from build123d import *

# Parameters (mm, degrees)
SKETCH1_R           = 0.5
BOSS_EXTRUDE1_DEPTH = 3
BOSS_EXTRUDE2_DEPTH = 3


with BuildPart() as part:
    # Sketch1 → Boss-Extrude1 (new body)
    with BuildSketch(Plane(origin=(0, 0, 0), x_dir=(1, 0, 0), z_dir=(0, 1, 0))):
        with BuildLine():
            Line((50, 20), (-50, 20))
            ThreePointArc((-50, 20), (-70, 0), (-50, -20))
            Line((-50, -20), (50, -20))
            ThreePointArc((50, -20), (70, 0), (50, 20))
        make_face()
        with Locations(Location((-48.85, -16.15, 0), (0, 0, 270))):
            Circle(SKETCH1_R, mode=Mode.SUBTRACT)
        with BuildLine():
            ThreePointArc((-48.85, -12.65), (-48.35, -13.15), (-48.85, -13.65))
            ThreePointArc((-48.85, -13.65), (-49.35, -13.15), (-48.85, -12.65))
        make_face(mode=Mode.SUBTRACT)
        with BuildLine():
            ThreePointArc((-48.85, -9.65), (-48.35, -10.15), (-48.85, -10.65))
            ThreePointArc((-48.85, -10.65), (-49.35, -10.15), (-48.85, -9.65))
        make_face(mode=Mode.SUBTRACT)
        Polygon((-30, -10), (-30, 8.197224362), (-16.352081728, -0.901387819), align=None, mode=Mode.SUBTRACT)
        Polygon((-2.704163457, -10), (-24.591673087, -10), (-13.647918272, -2.704163457), align=None, mode=Mode.SUBTRACT)
        with Locations(Location((48.85, -16.15, 0), (0, 0, 270))):
            Circle(SKETCH1_R, mode=Mode.SUBTRACT)
        with BuildLine():
            ThreePointArc((48.85, -12.65), (49.35, -13.15), (48.85, -13.65))
            ThreePointArc((48.85, -13.65), (48.35, -13.15), (48.85, -12.65))
        make_face(mode=Mode.SUBTRACT)
        with BuildLine():
            ThreePointArc((48.85, -9.65), (49.35, -10.15), (48.85, -10.65))
            ThreePointArc((48.85, -10.65), (48.35, -10.15), (48.85, -9.65))
        make_face(mode=Mode.SUBTRACT)
        Polygon((24.591673087, -10), (2.704163457, -10), (13.647918272, -2.704163457), align=None, mode=Mode.SUBTRACT)
        Polygon((30, 8.197224362), (30, -10), (16.352081728, -0.901387819), align=None, mode=Mode.SUBTRACT)
        with Locations(Location((-65, 0, 0), (0, 0, 270))):
            Circle(SKETCH1_R, mode=Mode.SUBTRACT)
        with Locations(Location((-62, 0, 0), (0, 0, 270))):
            Circle(SKETCH1_R, mode=Mode.SUBTRACT)
        with Locations(Location((-59, 0, 0), (0, 0, 270))):
            Circle(SKETCH1_R, mode=Mode.SUBTRACT)
        with BuildLine():
            ThreePointArc((-44.85, 0), (-46.021572875, -2.828427125), (-48.85, -4))
            ThreePointArc((-48.85, -4), (-52.85, 0), (-48.85, 4))
            ThreePointArc((-48.85, 4), (-46.021572875, 2.828427125), (-44.85, 0))
        make_face(mode=Mode.SUBTRACT)
        with BuildLine():
            ThreePointArc((-38.2, 0), (-38.7, -0.5), (-39.2, 0))
            ThreePointArc((-39.2, 0), (-38.7, 0.5), (-38.2, 0))
        make_face(mode=Mode.SUBTRACT)
        with BuildLine():
            ThreePointArc((-35.2, 0), (-35.7, -0.5), (-36.2, 0))
            ThreePointArc((-36.2, 0), (-35.7, 0.5), (-35.2, 0))
        make_face(mode=Mode.SUBTRACT)
        with Locations(Location((-32.7, 0, 0), (0, 0, 270))):
            Circle(SKETCH1_R, mode=Mode.SUBTRACT)
        with BuildLine():
            ThreePointArc((-48.85, 10.65), (-48.35, 10.15), (-48.85, 9.65))
            ThreePointArc((-48.85, 9.65), (-49.35, 10.15), (-48.85, 10.65))
        make_face(mode=Mode.SUBTRACT)
        with BuildLine():
            ThreePointArc((-48.85, 13.65), (-48.35, 13.15), (-48.85, 12.65))
            ThreePointArc((-48.85, 12.65), (-49.35, 13.15), (-48.85, 13.65))
        make_face(mode=Mode.SUBTRACT)
        with Locations(Location((-48.85, 16.15, 0), (0, 0, 270))):
            Circle(SKETCH1_R, mode=Mode.SUBTRACT)
        Polygon((-27.295836543, 10), (27.295836543, 10), (13.647918272, 0.901387819), (1.5, 9), (1.5, 5.394448725), (10.943754815, -0.901387819), (1.5, -7.197224362), (1.5, -10), (-1.5, -10), (-1.5, -7.197224362), (-10.943754815, -0.901387819), (-1.5, 5.394448725), (-1.5, 9), (-13.647918272, 0.901387819), align=None, mode=Mode.SUBTRACT)
        with Locations(Location((32.7, 0, 0), (0, 0, 270))):
            Circle(SKETCH1_R, mode=Mode.SUBTRACT)
        with BuildLine():
            ThreePointArc((35.2, 0), (35.7, 0.5), (36.2, 0))
            ThreePointArc((36.2, 0), (35.7, -0.5), (35.2, 0))
        make_face(mode=Mode.SUBTRACT)
        with BuildLine():
            ThreePointArc((38.2, 0), (38.7, 0.5), (39.2, 0))
            ThreePointArc((39.2, 0), (38.7, -0.5), (38.2, 0))
        make_face(mode=Mode.SUBTRACT)
        with BuildLine():
            ThreePointArc((48.85, 4), (52.85, 0), (48.85, -4))
            ThreePointArc((48.85, -4), (46.021572875, -2.828427125), (44.85, 0))
            ThreePointArc((44.85, 0), (46.021572875, 2.828427125), (48.85, 4))
        make_face(mode=Mode.SUBTRACT)
        with Locations(Location((62, 0, 0), (0, 0, 270))):
            Circle(SKETCH1_R, mode=Mode.SUBTRACT)
        with Locations(Location((65, 0, 0), (0, 0, 270))):
            Circle(SKETCH1_R, mode=Mode.SUBTRACT)
        with BuildLine():
            ThreePointArc((48.85, 10.65), (49.35, 10.15), (48.85, 9.65))
            ThreePointArc((48.85, 9.65), (48.35, 10.15), (48.85, 10.65))
        make_face(mode=Mode.SUBTRACT)
        with BuildLine():
            ThreePointArc((48.85, 13.65), (49.35, 13.15), (48.85, 12.65))
            ThreePointArc((48.85, 12.65), (48.35, 13.15), (48.85, 13.65))
        make_face(mode=Mode.SUBTRACT)
        with Locations(Location((48.85, 16.15, 0), (0, 0, 270))):
            Circle(SKETCH1_R, mode=Mode.SUBTRACT)
    extrude(amount=BOSS_EXTRUDE1_DEPTH)

    # Sketch1<3> → Boss-Extrude2 (add)
    with BuildSketch(Plane(origin=(0, 0, 0), x_dir=(1, 0, 0), z_dir=(0, 1, 0))):
        Polygon((0, -10), (0, 10), (-1.5, 9), (-1.5, 5.394448725), (-1.5, -7.197224362), (-1.5, -10), align=None)
        Polygon((1.5, 9), (0, 10), (0, -10), (1.5, -10), (1.5, -7.197224362), (1.5, 5.394448725), align=None)
        Polygon((1.5, 10), (0, 10), (1.5, 9), align=None)
        Polygon((-1.5, 9), (0, 10), (-1.5, 10), align=None)
    extrude(amount=BOSS_EXTRUDE2_DEPTH)


solid = part.part
Design review of the part built by this model. Coordinates are the model's own, in mm. A direction names the side the tool comes from. Give positions to 0.01 mm unless a question says otherwise; leave off trailing zeros. Loops run counter-clockwise (first coordinate to the right, second up) from the corner with the lowest first, then second, coordinate; pieces in that order, holes last. Notation, with made-up numbers: M 14.5,42 L 39.5,42 A25 ccw 39.5,64 Z; hole C -37.5,54.5 d9. An arc over 180 degrees is marked long. Write item = value, one per line.
Q1. For faces 1 (the flat face through (7.659, 1.479, -4.894)), 2 (the flat face through (-1, 0, 0)), list the 3-axis set-ups (+Z, -Z, +X, -X, +Y, -Y) from which the entire face can be reached by the end or side of a thin tool; tool diameter is ignored.
Output values:
face_1 = +Y, -Y
face_2 = +Z, -Z, +X, -X, -Y
Q2. We need section B-B (y = 0.5). Count the separate pieces of the cut face and the enclosed holes in it, plus the area to 3 significant figures.
Output values:
separate_pieces = 1
enclosed_holes = 33
area = 4,360 mm^2
Q3. To check wall thickness, follow line 1 (X direction, y = 1.4, z = -10.15); line 2 (X direction, y = 1.7, z = 9); line 3 (X direction, y = 1.75, z = -13.15). State the ranges of each line that lie inside material, in increasing order. Write a range as [from, to].
Output values:
line_1 = [-67.23, -49.35], [-48.35, 48.35], [49.35, 67.23]
line_2 = [-67.86, -30], [-28.5, -23.09], [-4.2, 4.2], [23.09, 28.5], [30, 67.86]
line_3 = [-65.07, -49.35], [-48.35, 48.35], [49.35, 65.07]
Q4. Insertion check: pin 1 (1.5 mm diameter, centred on y = 0.5, z = -8, fed in from -X); pin 2 (1.1 mm diameter, centred on y = 1, z = -9.5, fed in from -X); pin 3 (1 mm diameter, centred on x = 55, y = 2, fed in from +Z). Each pin has a flat end and moves straight along its axis. Give the tip position at first contact, or say it passes through.
Output values:
pin_1 = -68.64
pin_2 = -67.89
pin_3 = 19.49
Q5. We need section C-C (x = 57.5). Give the boundary of the cut face in (y, z).
Output values:
outline = M 0,-18.54 L 3,-18.54 L 3,18.54 L 0,18.54 Z
Q6. We need section A-A (x = -19). Give the boundary of the cut face in (y, z).
Output values:
outline = M 0,-20 L 3,-20 L 3,-10 L 0,-10 Z; M 0,-4.47 L 3,-4.47 L 3,-0.86 L 0,-0.86 Z; M 0,2.67 L 3,2.67 L 3,6.27 L 0,6.27 Z; M 0,10 L 3,10 L 3,20 L 0,20 Z
Q7. Draft analysis for pull direction Z (two halves, no side actions). For faces 3 (the cylindrical face through (-70, 1, 0)), 4 (the flat face through (1, 1, -20)), 5 (the flat face through (-23.1, 1.5, 5.4)), state which applies: +Z half, -Z half, draft (parallel to the pull), parting line (faces both ways), or undercut.
Output values:
face_3 = parting line
face_4 = -Z half
face_5 = undercut
